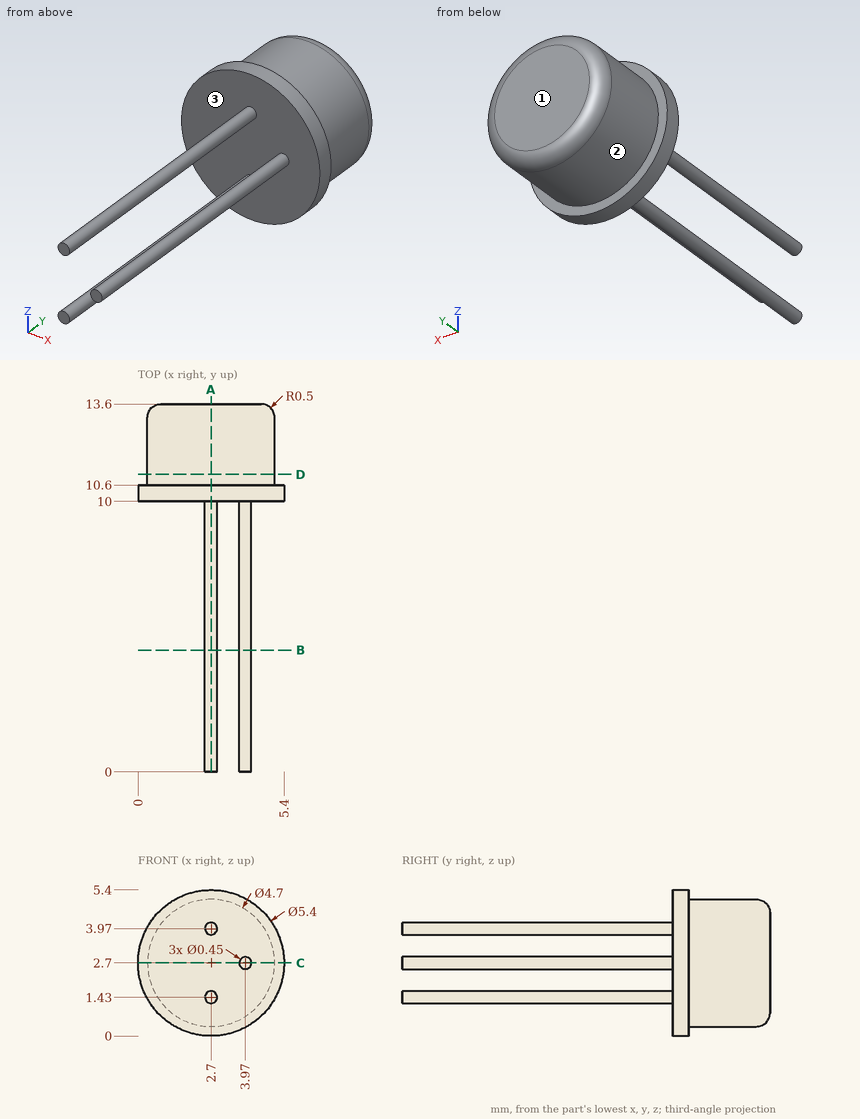
Study the drawing (mm; zero at the part's minimum x, y, z) and answer. A direction names the side the tool comes from. Give positions to 0.01 mm unless a question says otherwise; leave off trailing zeros. Order: outer loops, then holes, each group sorted by start corner. A loop starts at its lowest first (then second) coordinate and runs counter-clockwise, first axis right, second up. Notation, with made-up numbers: (-27, 32) - (9, 32) arc R15 ccw to (9, 53) - close; hole circle Ø3 at (-18, 62.5). An arc over 180 degrees is marked (long way). Use one line per item in the form item = value. Start each with the question number.
(1) A cutting plane is placed at B-B, the plane y = 4.5. Write down the section's boundary in (x, z) (3 decimals).
(2) Consider line 1 (Y direction, x = 0.85, z = 4.2); line 2 (Y direction, x = 1, z = 3.15); line 3 (X direction, y = 8.75, z = 2.75). Determine where each line is inside the solid, lowest interval first. Write a range as from..to.
(3) A cutting plane is placed at A-A, the plane x = 2.7. Write down the section's boundary in (y, z) (3 decimals).
(4) A cutting plane is placed at D-D, the plane y = 11. Write down the section's boundary in (x, z).
(5) Flat-ended cylindrical pins translate along their axes: pin 1 Ø2 at (x, z) = (3, 4.5) entering from -Y; pin 2 Ø1.5 at (x, y) = (2.5, 4) entering from -Z (3 decimals). Find the tip coordinate at first contact, or state that the pin passes through.
(6) A cutting plane is placed at C-C, the plane z = 2.7. Write down the section's boundary in (x, y) (3 decimals).
(7) For the marked faces 1, 2 and 3, determine the directions among +Z, -Z, +X, -X, +Y, -Y from which every point of the face is accessible in a straight line to the end or side of a thin tool.
Ans:
q1.outline = circle Ø0.45 at (2.7, 1.43); circle Ø0.45 at (2.7, 3.97); circle Ø0.45 at (3.97, 2.7)
q2.line_1 = 10..10.6
q2.line_2 = 10..13.6
q2.line_3 = 3.75..4.19
q3.outline = (0, 1.205) - (10, 1.205) - (10, 0) - (10.6, 0) - (10.6, 0.35) - (13.1, 0.35) arc R0.5 ccw to (13.6, 0.85) - (13.6, 4.55) arc R0.5 ccw to (13.1, 5.05) - (10.6, 5.05) - (10.6, 5.4) - (10, 5.4) - (10, 4.195) - (0, 4.195) - (0, 3.745) - (10, 3.745) - (10, 1.655) - (0, 1.655) - close
q4.outline = circle Ø4.7 at (2.7, 2.7)
q5.pin_1 = 0
q5.pin_2 = 1.205
q6.outline = (0, 10) - (3.745, 10) - (3.745, 0) - (4.195, 0) - (4.195, 10) - (5.4, 10) - (5.4, 10.6) - (5.05, 10.6) - (5.05, 13.1) arc R0.5 ccw to (4.55, 13.6) - (0.85, 13.6) arc R0.5 ccw to (0.35, 13.1) - (0.35, 10.6) - (0, 10.6) - close
q7.face_1 = +Z, -Z, +X, -X, +Y
q7.face_2 = +Y
q7.face_3 = -Y
